Work out the finished part from the listing and answer in its coordinate system (mm). A direction names the side the tool comes from. Give positions to 0.01 mm unless a question says otherwise; leave off trailing zeros. Write item = value, one per line. Start each with the question number.
1. The mould has two halves that part along X. Classify faces 1 (the face through (8.96, -3.17, 37.86)), 2 (the face through (6.825, 1.4, 8.6)), 3 (the face through (1.587, 0.035, 59.978)): released by +X, released by -X, zero draft, split by the parting line, or undercut.
2. For faces 4 (the face through (8.96, -3.17, 59.86)), 5 (the face through (0.606, 0.035, 58.413)), 6 (the face through (1.4, -1.4, 0)), determine the directions among +Z, -Z, +X, -X, +Y, -Y from which every point of the face is accessible in a straight line to the end or side of a thin tool.
3. Flat-ended cylindrical pins translate along their axes: pin 1 Ø3.5 at (y, z) = (0, 38) entering from +X (3 decimals); pin 2 Ø2.5 at (x, y) = (0, 0) entering from -Z (3 decimals); pin 3 Ø8 at (x, z) = (8.5, 23.5) entering from +Y; pin 4 Ø2.5 at (y, z) = (0, 10) entering from +X (3 decimals). Find the tip coordinate at first contact, or state that the pin passes through.
4. Section A-A on x = 6 is taken. Give the number of separate pieces and of enclosed holes in the cut face, plus the area to 3 significant figures.
5. Consider L1, parallel to Z at x = 6.5, y = 0 (1 decimal); L2, parallel to Z at x = 8, y = 0 (1 decimal); L3, parallel to Z at x = 7.5, y = -1. Determine where each line is inside the solid, lowest interval first. Write a range as [from, to].
Autodesk Inventor part; units mm, degrees
ref_plane "YZ Plane" through (0, 0, 0) normal (1, 0, 0) x (0, 1, 0)
ref_plane "XZ Plane" through (0, 0, 0) normal (0, 1, 0) x (-1, 0, 0)
ref_plane "XY Plane" through (0, 0, 0) normal (0, 0, 1) x (1, 0, 0)
sketch "Sketch1" plane through (0, 0, 0) normal (0, 0, 1) x (1, 0, 0)
  circle A0 centre (0, 0) radius 3.175
  circle A1 centre (0, 0) radius 1.5875
  dimension "d0" = 6.35
  dimension "d1" = 3.175
extrude "Extrusion1" add sketch "Sketch1" along normal blind 65
sketch "Sketch2" plane through (0, 0, 0) normal (1, 0, 0) x (0, 1, 0)
  circle A0 centre (0, 60) radius 3.175
  circle A1 centre (0, 60) radius 1.5875
  line L0 (3.175, 65) -> (-3.175, 65)
  circle A2 centre (0, 38) radius 3.175
  circle A3 centre (0, 38) radius 1.5875
  circle A4 centre (0, 10) radius 3.175
  circle A5 centre (0, 10) radius 1.5875
  point P0 (0, 0)
  dimension "d4" = 6.35
  dimension "d5" = 3.175
  dimension "d6" = 5
  dimension "d7" = 6.35
  dimension "d8" = 3.175
  dimension "d9" = 27
  dimension "d10" = 6.35
  dimension "d11" = 3.175
  dimension "d12" = 55
extrude "Extrusion2" add sketch "Sketch2" along normal blind 14.825 contours A0 | A2
extrude "Extrusion3" add sketch "Sketch2" along normal blind 6.825 contours A4
properties part number "Valve Tube"
Verdict:
q1.face_1 = zero draft
q1.face_2 = released by +X
q1.face_3 = undercut
q2.face_4 = +X
q2.face_5 = none
q2.face_6 = -Z, +X, -X, +Y, -Y
q3.pin_1 = 14.825
q3.pin_2 = 6.825
q3.pin_3 = through
q3.pin_4 = 3.175
q4.separate_pieces = 3
q4.enclosed_holes = 3
q4.area = 71.3 mm2
q5.L1 = [6.8, 8.4], [11.6, 13.2], [34.8, 36.4], [39.6, 41.2], [56.8, 58.4], [61.6, 63.2]
q5.L2 = [34.8, 36.4], [39.6, 41.2], [56.8, 58.4], [61.6, 63.2]
q5.L3 = [34.99, 36.77], [39.23, 41.01], [56.99, 58.77], [61.23, 63.01]
